Part model, mm, in its own coordinate system. Coordinates: 2 decimals unless noted, no trailing zeros. Loops run counter-clockwise (first coordinate to the right, second up) from the corner with the lowest first, then second, coordinate; pieces in that order, holes last. Notation, with made-up numbers: M -9,30 L 49,30 A28 ccw 49,59 Z; hole C 87,82.5 d6. An arc over 180 degrees is marked long. Answer as a JSON object with one key per item and string values. Group by question number.
1. Saw through at C-C on y = 4.25. Write the cut outline in (x, z).
2. Saw through at A-A on z = 1.55. Count the separate pieces of the cut face and the enclosed holes in it, then the cut area to 3 significant figures.
3. Drill centre lines: L1, parallel to Z at x = 10, y = 9.5; L2, parallel to X at y = 11.5, z = 0.3; L3, parallel to X at y = 12.5, z = 0.3. Where is each one in solid material? Low to high.
4. Drop flat-ended pins along their axis: pin 1 Ø0.5 at (y, z) = (5.5, 1.5) entering from +X; pin 2 Ø0.8 at (y, z) = (8.5, 1.5) entering from +X; pin 3 Ø0.8 at (x, z) = (6.5, 1.5) entering from +Y. Give the stop position or say it passes through.
5. Saw through at B-B on x = 27. Write the cut outline in (y, z), then the cut area to 3 significant figures.
from build123d import *

# Parameters (mm, degrees)
EXTRUDE_1_DEPTH = 1
EXTRUDE_2_DEPTH = 1


with BuildPart() as part:
    # 草图2 → 凸台-拉伸1 (new body)
    with BuildSketch(Plane.XY):
        Polygon((-20.5, 1), (39.75, 1), (39.75, 5.162511336), (38.191712307, 14), (-20.5, 14), align=None)
    extrude(amount=EXTRUDE_1_DEPTH)

    # 草图3 → 凸台-拉伸2 (add)
    # profile 1 of 2: a face of its own
    with BuildSketch(Plane.XY.offset(1)):
        with BuildLine():
            Line((10.481008306, 5.180393764), (11.248205137, 5.180393764))
            Line((11.248205137, 5.180393764), (11.248205137, 7.138792231))
            add(Edge.make_bspline(
                [(11.248205137, 7.138792231), (11.280268125, 7.133099507), (11.346316296, 7.121372777), (11.449283839, 7.111830081), (11.558346323, 7.105847724), (11.633053511, 7.105955746), (11.671485638, 7.106011317)],
                knots=[0, 0, 0, 0, 0.918585764, 1.892241272, 2.915691322, 4, 4, 4, 4], degree=3))
            add(Edge.make_bspline(
                [(11.671485638, 7.106011317), (11.729785366, 7.106041643), (11.845025321, 7.106101586), (12.015487029, 7.122104566), (12.181692953, 7.148109054), (12.343324735, 7.187087519), (12.50082336, 7.237455337), (12.654314168, 7.298636251), (12.80298521, 7.372843607), (12.946131503, 7.457876132), (13.080836859, 7.556007269), (13.198248856, 7.673392446), (13.300029776, 7.806147684), (13.3829419, 7.956216651), (13.450592093, 8.121964161), (13.499729538, 8.304167199), (13.533442208, 8.502261401), (13.541101546, 8.639948748), (13.545068751, 8.711264826)],
                knots=[0, 0, 0, 0, 1.003522523, 1.98364375, 2.944869411, 3.898614004, 4.843729631, 5.790462383, 6.741287792, 7.702146141, 8.655643954, 9.602935836, 10.551034771, 11.527201242, 12.5464735, 13.626777097, 14.770773406, 16, 16, 16, 16], degree=3))
            add(Edge.make_bspline(
                [(13.545068751, 8.711264826), (13.542621314, 8.767407479), (13.537856522, 8.876708825), (13.513966748, 9.035247709), (13.476887205, 9.183894353), (13.427758946, 9.323326261), (13.361987826, 9.451787215), (13.285822021, 9.571837482), (13.194736975, 9.681556892), (13.124181783, 9.745091174), (13.08871946, 9.77702466)],
                knots=[0, 0, 0, 0, 1.126595518, 2.193312949, 3.209115705, 4.196248007, 5.151139266, 6.097382339, 7.043709754, 8, 8, 8, 8], degree=3))
            add(Edge.make_bspline(
                [(13.08871946, 9.77702466), (13.048819299, 9.809220998), (12.967763644, 9.874626629), (12.829758648, 9.955555414), (12.678205789, 10.024206618), (12.512562725, 10.081265594), (12.332183639, 10.124461936), (12.1373955, 10.153402083), (11.928575344, 10.173362723), (11.784600384, 10.174930082), (11.710223363, 10.175739775)],
                knots=[0, 0, 0, 0, 0.838628006, 1.70364077, 2.610636308, 3.559859354, 4.568055018, 5.643200099, 6.782484425, 8, 8, 8, 8], degree=3))
            add(Edge.make_bspline(
                [(11.710223363, 10.175739775), (11.647547246, 10.17461434), (11.525326605, 10.172419704), (11.347031706, 10.166981234), (11.178493577, 10.158615294), (11.019779498, 10.147008031), (10.870704987, 10.134275133), (10.731447222, 10.118184966), (10.602269579, 10.099521255), (10.519709866, 10.084629366), (10.480064406, 10.07747823)],
                knots=[0, 0, 0, 0, 1.217605855, 2.374374404, 3.464660226, 4.494999595, 5.465333604, 6.370582827, 7.217548217, 8, 8, 8, 8], degree=3))
            Line((10.480064406, 10.07747823), (10.481008306, 5.180393764))
        make_face()
        with BuildLine():
            add(Edge.make_bspline(
                [(11.248205137, 9.536781383), (11.27774721, 9.542613746), (11.344633086, 9.555818735), (11.458986924, 9.567908637), (11.598601931, 9.577170189), (11.700441396, 9.579944465), (11.755574845, 9.581446392)],
                knots=[0, 0, 0, 0, 0.708180311, 1.603383121, 2.702528978, 4, 4, 4, 4], degree=3))
            add(Edge.make_bspline(
                [(11.755574845, 9.581446392), (11.793073561, 9.580660892), (11.86632842, 9.579126393), (11.973460101, 9.568908362), (12.074759776, 9.550753083), (12.17072877, 9.526581699), (12.260478405, 9.494387574), (12.34469003, 9.455320337), (12.422963445, 9.40924223), (12.495093205, 9.356007774), (12.560949572, 9.296684339), (12.618080877, 9.228947702), (12.666017981, 9.154020887), (12.706384443, 9.072744901), (12.737473184, 8.984178001), (12.75980904, 8.888502208), (12.77423784, 8.786014927), (12.776639324, 8.715407993), (12.777872842, 8.679140859)],
                knots=[0, 0, 0, 0, 1.164286524, 2.274468469, 3.33712435, 4.356941393, 5.343590938, 6.292901648, 7.23538906, 8.158502959, 9.072142365, 9.981112688, 10.900594105, 11.827687296, 12.792632354, 13.80775062, 14.873954761, 16, 16, 16, 16], degree=3))
            add(Edge.make_bspline(
                [(12.777872842, 8.679140859), (12.776613433, 8.640363707), (12.774167963, 8.56506781), (12.76019411, 8.455822494), (12.736174009, 8.3537626), (12.704419521, 8.258318665), (12.663824966, 8.169544292), (12.613156623, 8.088395241), (12.553144539, 8.014538438), (12.485007553, 7.946950655), (12.408057089, 7.887831849), (12.324594044, 7.835136167), (12.233012254, 7.791830384), (12.134562282, 7.756148342), (12.029100063, 7.727426213), (11.916122917, 7.708209363), (11.796164858, 7.695683181), (11.713720416, 7.693741042), (11.671485638, 7.692746119)],
                knots=[0, 0, 0, 0, 1.10647952, 2.148516939, 3.135813804, 4.093347323, 5.013956832, 5.913991464, 6.814877829, 7.723438285, 8.645449828, 9.577866136, 10.534345172, 11.529217628, 12.562346088, 13.648092354, 14.795160789, 16, 16, 16, 16], degree=3))
            add(Edge.make_bspline(
                [(11.671485638, 7.692746119), (11.63021482, 7.692200684), (11.551388911, 7.691158922), (11.439442024, 7.698169967), (11.339043734, 7.709168238), (11.277392814, 7.723672298), (11.248205137, 7.730539021)],
                knots=[0, 0, 0, 0, 1.161518353, 2.218461969, 3.156558288, 4, 4, 4, 4], degree=3))
            Line((11.248205137, 7.730539021), (11.248205137, 9.536781383))
        make_face(mode=Mode.SUBTRACT)
    # profile 2 of 2: a face of its own
    with BuildSketch(Plane.XY.offset(1)):
        with BuildLine():
            Line((9.494613566, 10.144699032), (8.727416734, 10.144699032))
            Line((8.727416734, 10.144699032), (8.727416734, 7.120977159))
            add(Edge.make_bspline(
                [(8.727416734, 7.120977159), (8.72570679, 7.061167821), (8.722407633, 6.945772013), (8.709631742, 6.778889408), (8.688170718, 6.624510706), (8.658230337, 6.482310653), (8.619760507, 6.352261672), (8.572739739, 6.23481111), (8.517630595, 6.129485265), (8.454448576, 6.036324521), (8.382626209, 5.95552631), (8.305148113, 5.884790711), (8.220215209, 5.826242463), (8.129699085, 5.776987395), (8.031964883, 5.740430268), (7.92791034, 5.715069684), (7.817708054, 5.699600995), (7.742020532, 5.698067043), (7.703230938, 5.697280898)],
                knots=[0, 0, 0, 0, 1.442558911, 2.783265207, 4.033293762, 5.19797452, 6.283894868, 7.299176403, 8.243481286, 9.144954945, 10.005756174, 10.844503658, 11.66816234, 12.486940923, 13.323278702, 14.176003432, 15.065208066, 16, 16, 16, 16], degree=3))
            add(Edge.make_bspline(
                [(7.703230938, 5.697280898), (7.667274667, 5.697698259), (7.596903954, 5.698515082), (7.494090027, 5.713985225), (7.396870282, 5.740714967), (7.304631521, 5.777818192), (7.21742606, 5.824889909), (7.136059616, 5.88355453), (7.060255296, 5.953212566), (6.989139578, 6.033370677), (6.925239634, 6.126225718), (6.869986093, 6.231342171), (6.822149712, 6.348958788), (6.784585577, 6.479350068), (6.752971554, 6.621900529), (6.730985424, 6.776989679), (6.716631756, 6.944497921), (6.714275141, 7.060313631), (6.713056908, 7.120183655)],
                knots=[0, 0, 0, 0, 0.880869997, 1.723967724, 2.54076827, 3.348096003, 4.15667844, 4.964596865, 5.80091263, 6.676282017, 7.586647838, 8.557371955, 9.582678263, 10.694376867, 11.880403812, 13.160330013, 14.532054847, 16, 16, 16, 16], degree=3))
            Line((6.713056908, 7.120183655), (6.713056908, 10.144699032))
            Line((6.713056908, 10.144699032), (5.945860076, 10.144699032))
            Line((5.945860076, 10.144699032), (5.945860076, 7.166692176))
            add(Edge.make_bspline(
                [(5.945860076, 7.166692176), (5.947811599, 7.077745647), (5.951582552, 6.905873082), (5.976446082, 6.658325939), (6.014608186, 6.430215629), (6.067172501, 6.221450241), (6.133738874, 6.031572757), (6.214969708, 5.861101508), (6.31051972, 5.710146918), (6.421501903, 5.57950536), (6.544430093, 5.46706325), (6.67617651, 5.36843753), (6.819480172, 5.287205614), (6.971797177, 5.219666165), (7.13441307, 5.168482563), (7.306791456, 5.134357698), (7.4884993, 5.112474089), (7.613091953, 5.111823473), (7.676775907, 5.111490919)],
                knots=[0, 0, 0, 0, 1.389947096, 2.68581329, 3.884176986, 5.001519278, 6.046082896, 7.023506491, 7.946473535, 8.830015835, 9.69383004, 10.545329235, 11.396344648, 12.262399475, 13.145009074, 14.054291982, 15.00547603, 16, 16, 16, 16], degree=3))
            add(Edge.make_bspline(
                [(7.676775907, 5.111490919), (7.743278786, 5.112273586), (7.873172166, 5.113802291), (8.063018751, 5.134646007), (8.242559022, 5.17174834), (8.412356909, 5.222999832), (8.571712956, 5.292121054), (8.721258262, 5.375818025), (8.860035095, 5.476399667), (8.989854742, 5.590728631), (9.106884057, 5.723770561), (9.2085838, 5.876673755), (9.294366864, 6.048926123), (9.364814239, 6.239771985), (9.420601689, 6.449185846), (9.460084235, 6.67781481), (9.487297433, 6.925232139), (9.491500008, 7.096800861), (9.493669666, 7.185376411)],
                knots=[0, 0, 0, 0, 1.013962662, 1.980471211, 2.907472823, 3.806985122, 4.680561309, 5.551651082, 6.415505808, 7.289926821, 8.185106327, 9.109702809, 10.082849364, 11.113391155, 12.207519227, 13.383461846, 14.649163417, 16, 16, 16, 16], degree=3))
            Line((9.493669666, 7.185376411), (9.494613566, 10.144699032))
        make_face()
    extrude(amount=EXTRUDE_2_DEPTH)


solid = part.part
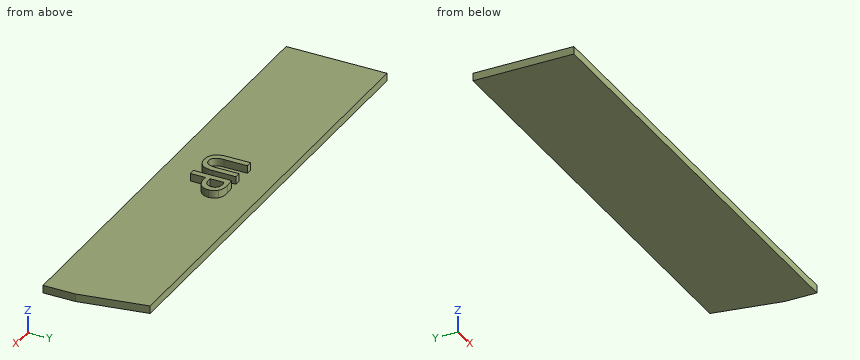
Outcome:
{
 "1": {"outline": "M -20.5,0 L 39.75,0 L 39.75,1 L -20.5,1 Z"},
 "2": {"separate pieces": "2", "enclosed holes": "1", "area": "15.4 mm²"},
 "3": {"L1": "z = 0 to 1", "L2": "x = -20.5 to 38.63", "L3": "x = -20.5 to 38.46"},
 "4": {"pin 1": "stops at x = 11.25", "pin 2": "stops at x = 13.55", "pin 3": "stops at y = 10.14"},
 "5": {"outline": "M 1,0 L 14,0 L 14,1 L 1,1 Z", "area": "13.0 mm²"}
}
